```python
from build123d import *

# Parameters (mm, degrees)
BOSS_EXTRUDE1_DEPTH = 14
BOSS_EXTRUDE2_DEPTH = 4
SKETCH3_R           = 2
CUT_EXTRUDE1_DEPTH  = 4


with BuildPart() as part:
    # Sketch1 → Boss-Extrude1 (new body)
    with BuildSketch(Plane.XY):
        Polygon((0, 0), (0, 38), (4, 38), (4, 4), (38, 4), (38, 0), align=None)
    extrude(amount=BOSS_EXTRUDE1_DEPTH)

    # Sketch2 → Boss-Extrude2 (add)
    with BuildSketch(Plane(origin=(0, 0, 0), x_dir=(-1, 0, 0), z_dir=(0, 0, -1))):
        Polygon((-4, 38), (-38, 4), (-4, 4), align=None)
        Polygon((-38, 4), (-38, 0), (0, 0), (0, 38), (-4, 38), (-4, 4), align=None)
    extrude(amount=BOSS_EXTRUDE2_DEPTH)

    # Sketch3 → Cut-Extrude1 (cut)
    with BuildSketch(Plane(origin=(4, 0, 0), x_dir=(0, 0, -1), z_dir=(1, 0, 0))):
        with Locations(Location((-5, 30.38, 0), (0, 0, 90))):
            Circle(SKETCH3_R)
        with Locations(Location((-5, 12.6, 0), (0, 0, 90))):
            Circle(SKETCH3_R)
    cut_extrude1 = extrude(amount=-CUT_EXTRUDE1_DEPTH, mode=Mode.SUBTRACT)

    # Mirror4: Cut-Extrude1 across plane
    add(cut_extrude1.mirror(Plane(origin=(0, 0, 0), x_dir=(0, 0, 1), z_dir=(0.7071067811865438, -0.7071067811865512, 0))), mode=Mode.SUBTRACT)


solid = part.part
```
Check sheet for the modelled part. Datum: model origin and axes. Units: mm. A direction names the side the tool comes from. Round coordinates to 2 decimals unless told otherwise and drop trailing zeros. Loops run counter-clockwise (first coordinate to the right, second up) from the corner with the lowest first, then second, coordinate; pieces in that order, holes last. Notation, with made-up numbers: (56, 81.5) - (105, 81.5) arc R29 cw to (105, 107.5) - close; hole circle Ø8 at (81.25, 83). An arc over 180 degrees is marked (long way). Answer as a JSON object with one key per item and string values. Group by question number.
Q1. Sectioned sample at C-C, the plane y = 12.6. Enter the section's corners in (x, z).
Q2. Mould release check, pull along Z, two halves, no side actions. Record for faces 3 (the face through (0, 19, 5)), 4 (the face through (15, 15, -4)), 5 (the face through (2.028, 28.382, 5.088)), 6 (the face through (11.126, 2.028, 6.352)): released by +Z, released by -Z, zero draft, split by the parting line, or undercut.
Q3. Sectioned sample at A-A, the plane x = 30.38. Enter the section's corners in (y, z), plus the area to 3 significant figures.
Q4. Sectioned sample at D-D, the plane x = 18. Enter the section's corners in (y, z).
Q5. Sectioned sample at B-B, the plane z = 5. Enter the section's corners in (x, y).
Q6. Scan lines: line 1 along Z through (x, y) = (30.38, 2.1); line 2 along Y through (x, z) = (6, 5.5). Record each from-to range of solid material in increasing order. Write a range as [from, to].
Q7. Set-up check for faces 1 (the face through (14, 14, 0)), 2 (the face through (2, 38, 5)): record each of +Z, -Z, +X, -X, +Y, -Y from which the full face is reachable in a straight line by a thin tool's end or side.
Q8. Gauge pin test, flat ends, axial feed: P1, Ø3, axis at y = 19.5, z = 5.5, coming from the +X side; P2, Ø3.5, axis at y = 30.38, z = 5, coming from the -X side; P3, Ø7, axis at x = 19, z = 9, coming from the +Y side; P4, Ø1, axis at y = 10, z = -1.5, coming from the +X side. Record the tip position at first contact, or that the pin passes through.
Solution:
{
 "1": {"outline": "(0, -4) - (29.4, -4) - (29.4, 0) - (4, 0) - (4, 3) - (0, 3) - close; (0, 7) - (4, 7) - (4, 14) - (0, 14) - close"},
 "2": {"face 3": "zero draft", "face 4": "released by -Z", "face 5": "undercut", "face 6": "undercut"},
 "3": {"outline": "(0, -4) - (11.62, -4) - (11.62, 0) - (4, 0) - (4, 3) - (0, 3) - close; (0, 7) - (4, 7) - (4, 14) - (0, 14) - close", "area": "86.5 mm²"},
 "4": {"outline": "(0, -4) - (24, -4) - (24, 0) - (4, 0) - (4, 14) - (0, 14) - close"},
 "5": {"outline": "(0, 0) - (10.6, 0) - (10.6, 4) - (4, 4) - (4, 10.6) - (0, 10.6) - close; (0, 14.6) - (4, 14.6) - (4, 28.38) - (0, 28.38) - close; (0, 32.38) - (4, 32.38) - (4, 38) - (0, 38) - close; (14.6, 0) - (28.38, 0) - (28.38, 4) - (14.6, 4) - close; (32.38, 0) - (38, 0) - (38, 4) - (32.38, 4) - close"},
 "6": {"line 1": "z = [-4, 3], [7, 14]", "line 2": "y = [0, 4]"},
 "7": {"face 1": "+Z, +X, +Y", "face 2": "+Z, -Z, +X, -X, +Y"},
 "8": {"P1": "stops at x = 4", "P2": "passes through", "P3": "stops at y = 4", "P4": "stops at x = 32.5"}
}
